For this review, take the finished solid that the model builds, in its own axes (mm). Face numbers are marked on the shaded views. A direction names the side the tool comes from. Round coordinates to 2 decimals unless told otherwise and drop trailing zeros. Loops run counter-clockwise (first coordinate to the right, second up) from the corner with the lowest first, then second, coordinate; pieces in that order, holes last. Notation, with made-up numbers: (-27.5, -13) -> (-5.5, -13) arc R14 ccw to (-5.5, -1) -> close; hole circle Ø5 at (25, 65.5). An arc over 180 degrees is marked (long way). Write each question's results on one line, items separated by ' | '.
```python
from build123d import *

# Parameters (mm, degrees)
EXTRUDE_1_DEPTH     = 1
SKETCH_2_W          = 1.2
SKETCH_2_H          = 13.45
SKETCH_2_H_2        = 9.3
EXTRUDE_2_DEPTH     = 7
CUT_EXTRUDE_1_REACH = 29.95
SKETCH_3_W          = 7
SKETCH_3_H          = 7
CUT_EXTRUDE_2_REACH = 29.95
SKETCH_4_W          = 7
SKETCH_4_H          = 3.5
FILLET_1_R          = 0.3


with BuildPart() as part:
    # 草图1 → 凸台-拉伸1 (new body)
    with BuildSketch(Plane.XY):
        with BuildLine():
            Line((2, 0), (28.95, 0))
            ThreePointArc((28.95, 0), (30.364213562, 0.585786438), (30.95, 2))
            Line((30.95, 2), (30.95, 11.45))
            ThreePointArc((30.95, 11.45), (30.364213562, 12.864213562), (28.95, 13.45))
            Line((28.95, 13.45), (2, 13.45))
            ThreePointArc((2, 13.45), (0.585786438, 12.864213562), (0, 11.45))
            Line((0, 11.45), (0, 2))
            ThreePointArc((0, 2), (0.585786438, 0.585786438), (2, 0))
        make_face()
    extrude(amount=EXTRUDE_1_DEPTH)

    # 草图2 → 凸台-拉伸2 (add)
    with BuildSketch(Plane.XY.offset(1)):
        with Locations((27.35, 6.725)):
            Rectangle(SKETCH_2_W, SKETCH_2_H)
        with Locations((3.6, 6.725)):
            Rectangle(SKETCH_2_W, SKETCH_2_H_2)
    extrude(amount=EXTRUDE_2_DEPTH)

    # 草图3 → 切除-拉伸1 (cut, up to next)
    with BuildSketch(Plane(origin=(27.95, 0, 0), x_dir=(0, 0, -1), z_dir=(1, 0, 0)), mode=Mode.PRIVATE) as cut_extrude_1_sk1:
        with Locations((-4.5, 6.725)):
            Rectangle(SKETCH_3_W, SKETCH_3_H)
    cut_extrude_1_tool1 = extrude(cut_extrude_1_sk1.sketch, amount=-CUT_EXTRUDE_1_REACH, mode=Mode.PRIVATE) & part.part
    add(cut_extrude_1_tool1.solids().sort_by_distance((27.95, 6.725, 4.5))[0], mode=Mode.SUBTRACT)

    # 草图4 → 切除-拉伸2 (cut, up to next)
    with BuildSketch(Plane.ZY.offset(-3), mode=Mode.PRIVATE) as cut_extrude_2_sk1:
        with Locations((4.5, 6.725)):
            Rectangle(SKETCH_4_W, SKETCH_4_H)
    cut_extrude_2_tool1 = extrude(cut_extrude_2_sk1.sketch, amount=-CUT_EXTRUDE_2_REACH, mode=Mode.PRIVATE) & part.part
    add(cut_extrude_2_tool1.solids().sort_by_distance((3, 6.725, 4.5))[0], mode=Mode.SUBTRACT)

    # 圆角1
    fillet_1_edges = [part.edges().sort_by_distance(p)[0] for p in [
        (26.75, 11.8375, 8),
        (27.35, 0, 8),
        (27.95, 1.6125, 8),
        (27.35, 13.45, 8),
        (3, 9.925, 8),
        (3.6, 2.075, 8),
        (4.2, 3.525, 8),
        (3.6, 11.375, 8),
        (26.75, 1.6125, 8),
        (27.95, 11.8375, 8),
        (27.35, 3.225, 8),
        (27.35, 10.225, 8),
        (3, 3.525, 8),
        (4.2, 9.925, 8),
        (3.6, 8.475, 8),
        (3.6, 4.975, 8),
    ]]
    fillet(fillet_1_edges, radius=FILLET_1_R)


solid = part.part
```
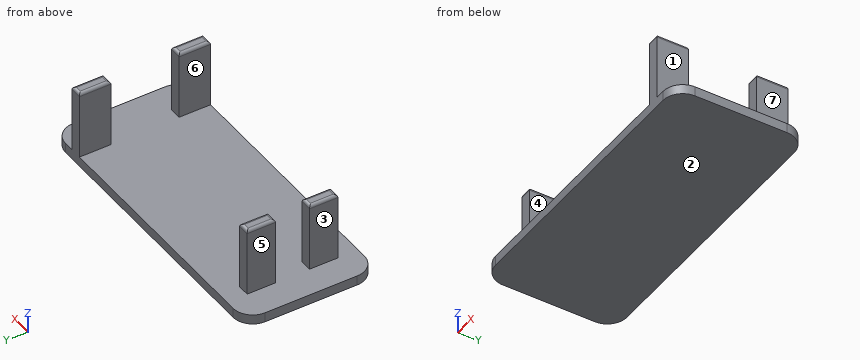
1. Consider section A-A (z = 5). State the section outline as (x, y) points (3 decimals).
Values found:
outline: (3, 2.075) -> (4.2, 2.075) -> (4.2, 4.975) -> (3, 4.975) -> close; (3, 8.475) -> (4.2, 8.475) -> (4.2, 11.375) -> (3, 11.375) -> close; (26.75, 0) -> (27.95, 0) -> (27.95, 3.225) -> (26.75, 3.225) -> close; (26.75, 10.225) -> (27.95, 10.225) -> (27.95, 13.45) -> (26.75, 13.45) -> close
2. Consider section B-B (y = 9.5). State the section outline as (x, z) points, plus the area to 3 significant figures.
Values found:
outline: (0, 0) -> (30.95, 0) -> (30.95, 1) -> (4.2, 1) -> (4.2, 7.7) arc R0.3 ccw to (3.9, 8) -> (3.3, 8) arc R0.3 ccw to (3, 7.7) -> (3, 1) -> (0, 1) -> close | area: 39.3 mm2
3. Consider section C-C (x = 14.5). State the section outline as (y, z) points, plus the area to 4 significant figures.
Values found:
outline: (0, 0) -> (13.45, 0) -> (13.45, 1) -> (0, 1) -> close | area: 13.45 mm2
4. For pin 1 (2.5 mm diameter, centred on y = 9.5, z = 5, fed in from +X); pin 2 (1.3 mm diameter, centred on x = 4, z = 4.5, fed in from +Y) (3 decimals); pin 3 (3 mm diameter, centred on y = 10, z = 4.5, fed in from -X), all flat-tipped, find the tip position at first contact; note any pin that passes through.
Values found:
pin 1: stops at x = 27.95 | pin 2: stops at y = 11.375 | pin 3: stops at x = 3
5. Draft analysis for pull direction X (two halves, no side actions). For the marked faces 5, 6 and 7, state which applies: released by +X, released by -X, zero draft, split by the parting line, or undercut.
Values found:
face 5: released by -X | face 6: undercut | face 7: released by +X
6. To check wall thickness, follow probe 1 along X at (y, z) = (11, 7); probe 2 along X at (y, z) = (10, 4); probe 3 along X at (y, z) = (12.25, 2). State the ranges of each line that lie inside material, in increasing order.
Values found:
probe 1: x = 3 to 4.2, 26.75 to 27.95 | probe 2: x = 3 to 4.2 | probe 3: x = 26.75 to 27.95
7. Tool access review of the marked faces 1, 2, 3 and 4: name each direction out of +Z, -Z, +X, -X, +Y, -Y from which nothing blocks a thin tool from reaching the whole face with its end or side.
Values found:
face 1: +Z, +X, +Y, -Y | face 2: -Z, +X, -X, +Y, -Y | face 3: +Z, -X, +Y, -Y | face 4: +Z, +Y, -Y
8. Consider section D-D (y = 12.5). State the section outline as (x, z) points.
Values found:
outline: (0.3, 0) -> (30.65, 0) -> (30.65, 1) -> (27.95, 1) -> (27.95, 7.7) arc R0.3 ccw to (27.65, 8) -> (27.05, 8) arc R0.3 ccw to (26.75, 7.7) -> (26.75, 1) -> (0.3, 1) -> close
